from build123d import *

# Parameters (mm, degrees)
SKETCH_1_W          = 280
SKETCH_1_H          = 390
EXTRUDE_1_DEPTH     = 3
SKETCH_2_R          = 1.5
CUT_EXTRUDE_1_DEPTH = 481.113528241
SKETCH_3_R          = 1.5
CUT_EXTRUDE_2_DEPTH = 481.113528241
CUT_EXTRUDE_5_DEPTH = 481.113528241
SKETCH_7_W          = 5
SKETCH_7_H          = 25
CUT_EXTRUDE_6_DEPTH = 481.113528241


with BuildPart() as part:
    # 草图1 → 凸台-拉伸1 (new body)
    with BuildSketch(Plane(origin=(0, 0, 0), x_dir=(1, 0, 0), z_dir=(0, 1, 0))):
        with Locations((140, 195)):
            Rectangle(SKETCH_1_W, SKETCH_1_H)
    extrude(amount=EXTRUDE_1_DEPTH)

    # 草图2 → 切除-拉伸1 (cut, through all)
    with BuildSketch(Plane(origin=(0, 3, 0), x_dir=(1, 0, 0), z_dir=(0, 1, 0))):
        with Locations(Location((140, 383, 0), (0, 0, 270))):
            Circle(SKETCH_2_R)
        with Locations(Location((140, 334, 0), (0, 0, 270))):
            Circle(SKETCH_2_R)
        with Locations(Location((264.5, 383, 0), (0, 0, 270))):
            Circle(SKETCH_2_R)
        with Locations(Location((264.5, 334, 0), (0, 0, 270))):
            Circle(SKETCH_2_R)
        with Locations(Location((15.5, 383, 0), (0, 0, 90))):
            Circle(SKETCH_2_R)
        with Locations(Location((15.5, 334, 0), (0, 0, 90))):
            Circle(SKETCH_2_R)
        with Locations(Location((264.5, 56, 0), (0, 0, 90))):
            Circle(SKETCH_2_R)
        with Locations(Location((264.5, 7, 0), (0, 0, 90))):
            Circle(SKETCH_2_R)
        with Locations(Location((140, 7, 0), (0, 0, 90))):
            Circle(SKETCH_2_R)
        with Locations(Location((140, 56, 0), (0, 0, 90))):
            Circle(SKETCH_2_R)
        with Locations(Location((15.5, 56, 0), (0, 0, 270))):
            Circle(SKETCH_2_R)
        with Locations(Location((15.5, 7, 0), (0, 0, 270))):
            Circle(SKETCH_2_R)
    extrude(amount=-CUT_EXTRUDE_1_DEPTH, mode=Mode.SUBTRACT)

    # 草图3 → 切除-拉伸2 (cut, through all)
    with BuildSketch(Plane(origin=(0, 3, 0), x_dir=(1, 0, 0), z_dir=(0, 1, 0))):
        with Locations(Location((117, 211.5, 0), (0, 0, 270))):
            Circle(SKETCH_3_R)
        with Locations(Location((163, 211.5, 0), (0, 0, 270))):
            Circle(SKETCH_3_R)
        with Locations(Location((163, 178.5, 0), (0, 0, 270))):
            Circle(SKETCH_3_R)
        with Locations(Location((117, 178.5, 0), (0, 0, 270))):
            Circle(SKETCH_3_R)
    extrude(amount=-CUT_EXTRUDE_2_DEPTH, mode=Mode.SUBTRACT)

    # 草图6 → 切除-拉伸5 (cut, through all)
    with BuildSketch(Plane(origin=(0, 3, 0), x_dir=(1, 0, 0), z_dir=(0, 1, 0))):
        with BuildLine():
            Line((121, 211.5), (159, 211.5))
            ThreePointArc((159, 211.5), (160.171572875, 208.671572875), (163, 207.5))
            Line((163, 207.5), (163, 182.5))
            ThreePointArc((163, 182.5), (160.171572875, 181.328427125), (159, 178.5))
            Line((159, 178.5), (121, 178.5))
            ThreePointArc((121, 178.5), (119.828427125, 181.328427125), (117, 182.5))
            Line((117, 182.5), (117, 207.5))
            ThreePointArc((117, 207.5), (119.828427125, 208.671572875), (121, 211.5))
        make_face()
    extrude(amount=-CUT_EXTRUDE_5_DEPTH, mode=Mode.SUBTRACT)

    # 草图7 → 切除-拉伸6 (cut, through all)
    with BuildSketch(Plane(origin=(0, 3, 0), x_dir=(1, 0, 0), z_dir=(0, 1, 0))):
        with Locations((165.5, 195)):
            Rectangle(SKETCH_7_W, SKETCH_7_H)
    extrude(amount=-CUT_EXTRUDE_6_DEPTH, mode=Mode.SUBTRACT)


solid = part.part
Check sheet for the modelled part. Datum: model origin and axes. Units: mm. Give positions to 0.01 mm unless a question says otherwise; leave off trailing zeros. Answer as a JSON object with one key per item and string values. Group by question number.
Q1. Material ranges on line 1 along X through (y, z) = (1.95, -383); line 2 along Z through (x, y) = (163, 2.2); line 3 along Z through (x, y) = (140, 1.5), recorded low to high. Write a range as [from, to].
Q2. Cross-section at A-A on y = 2.25. Give the number of separate pieces and of enclosed holes in the cut face, then the cut area to 3 significant figures.
Q3. Go/stop test with a flat-tipped pin: P1, Ø1.8, axis at x = 264.5, z = -7, coming from the +Y side. Record where the tip stops, or that it passes through.
Evaluation:
{
 "1": {"line 1": "x = [0, 14], [17, 138.5], [141.5, 263], [266, 280]", "line 2": "z = [-390, -213], [-210, -207.5], [-182.5, -180], [-177, 0]", "line 3": "z = [-390, -384.5], [-381.5, -335.5], [-332.5, -211.5], [-178.5, -57.5], [-54.5, -8.5], [-5.5, 0]"},
 "2": {"separate pieces": "1", "enclosed holes": "17", "area": "107,000 mm2"},
 "3": {"P1": "passes through"}
}
